Autodesk Inventor part; units mm, degrees
ref_plane "YZ Plane" through (0, 0, 0) normal (1, 0, 0) x (0, 1, 0)
ref_plane "XZ Plane" through (0, 0, 0) normal (0, 1, 0) x (-1, 0, 0)
ref_plane "XY Plane" through (0, 0, 0) normal (0, 0, 1) x (1, 0, 0)
sketch "Sketch1" plane through (0, 0, 0) normal (0, 0, 1) x (1, 0, 0)
  line L0 (-20, -20) -> (20, -20)
  line L1 (20, -20) -> (20, 20)
  line L2 (20, 20) -> (-20, 20)
  line L3 (-20, 20) -> (-20, -20)
  line L4 (-20, -20) -> (20, 20) construction
  line L5 (20, -20) -> (-20, 20) construction
  point P0 (0, 0)
  dimension "d0" = 40
  dimension "d1" = 40
extrude "Extrusion1" add sketch "Sketch1" along normal blind 10
sketch "Sketch2" plane through (0, 0, 10) normal (0, 0, 1) x (1, 0, 0)
  circle A0 centre (-14, 14) radius 1.05
  circle A1 centre (-14, -14) radius 1.05
  circle A2 centre (14, -14) radius 1.05
  circle A3 centre (14, 14) radius 1.05
  point P0 (0, 0)
  dimension "d4" = 2.1
  dimension "d5" = 2.1
  dimension "d6" = 2.1
  dimension "d7" = 2.1
  dimension "d8" = 14
  dimension "d9" = 14
  dimension "d10" = 14
  dimension "d11" = 14
extrude "Extrusion2" cut sketch "Sketch2" against normal blind 10
sketch "Sketch3" plane through (0, 0, 10) normal (0, 0, 1) x (1, 0, 0)
  line L0 (-7.5, -18) -> (7.5, -18)
  line L1 (7.5, -18) -> (7.5, -10)
  line L2 (7.5, -10) -> (-7.5, -10)
  line L3 (-7.5, -10) -> (-7.5, -18)
  line L4 (-7.5, -18) -> (7.5, -10) construction
  line L5 (7.5, -18) -> (-7.5, -10) construction
  point P0 (0, 0)
  point P1 (0, -14)
  dimension "d14" = 15
  dimension "d15" = 8
  dimension "d16" = 14
extrude "Extrusion3" cut sketch "Sketch3" against normal blind 10
sketch "Sketch4" plane through (-20, -20, 0) normal (0, -1, 0) x (1, 0, 0)
  line L0 (0, 0) -> (-10, 0)
  line L1 (-10, 0) -> (-10, 10)
  line L2 (-10, 10) -> (0, 10)
  line L3 (0, 10) -> (0, 0)
  line L4 (50, 0) -> (40, 0)
  line L5 (40, 0) -> (40, 10)
  line L6 (40, 10) -> (50, 10)
  line L7 (50, 10) -> (50, 0)
  line L8 (0, 0) -> (0, 10)
  line L9 (40, 0) -> (40, 10)
  line L10 (0, 0) -> (40, 0)
  line L11 (0, 10) -> (40, 10)
  point P0 (20, 0)
  dimension "d19" = 10
  dimension "d20" = 10
extrude "Extrusion4" add sketch "Sketch4" against normal blind 5 contours L0 L1 L2 L3 | L5 L6 L7 L4
sketch "Sketch5" plane through (-20, -15, 0) normal (0, 1, 0) x (1, 0, 0)
  circle A0 centre (-5, -5) radius 2.05
  circle A1 centre (45, -5) radius 2.05
  line L0 (-10, 0) -> (-10, -10)
  line L1 (-10, -10) -> (0, -10)
  line L2 (50, 0) -> (40, 0)
  line L3 (50, -10) -> (50, 0)
  point P0 (20, 0)
  dimension "d23" = 4.1
  dimension "d24" = 4.1
  dimension "d25" = 5
  dimension "d26" = 5
  dimension "d27" = 5
  dimension "d28" = 5
extrude "Extrusion5" cut sketch "Sketch5" against normal blind 5
sketch "Sketch6" plane through (-20, 20, 0) normal (0, 1, 0) x (1, 0, 0)
  line L0 (30, -10) -> (10, -10)
  line L1 (10, -10) -> (10, 0)
  line L2 (10, 0) -> (30, 0)
  line L3 (30, 0) -> (30, -10)
  line L4 (40, -10) -> (0, -10)
  line L5 (40, 0) -> (40, -10)
  line L6 (40, 0) -> (0, 0)
  line L7 (0, 0) -> (0, -10)
  point P0 (20, 0)
  dimension "d33" = 20
  dimension "d34" = 10
extrude "Extrusion6" add sketch "Sketch6" along normal blind 32 contours L0 L1 L2 L3
sketch "Sketch7" plane through (0, 0, 0) normal (0, 0, -1) x (-1, 0, 0)
  circle A0 centre (-7.5, 49.5) radius 1.05
  circle A1 centre (-7.5, 22.5) radius 1.05
  circle A2 centre (7.5, 49.5) radius 1.05
  circle A3 centre (7.5, 22.5) radius 1.05
  line L0 (-10, 52) -> (10, 52)
  line L1 (-10, 20) -> (-10, 52)
  point P0 (0, 0)
  dimension "d35" = 2.1
  dimension "d36" = 2.1
  dimension "d37" = 2.1
  dimension "d38" = 2.1
  dimension "d39" = 15
  dimension "d40" = 27
  dimension "d41" = 2.5
  dimension "d42" = 2.5
extrude "Extrusion7" cut sketch "Sketch7" against normal blind 32
properties part number "camera_new"
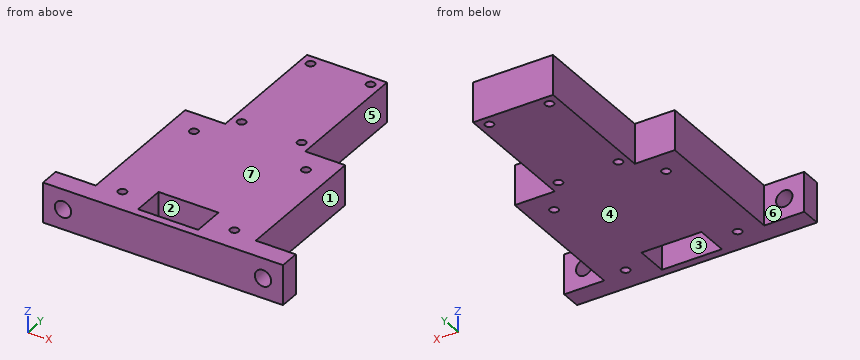
Design review of the part built by this model. Coordinates are the model's own, in mm. Face numbers are marked on the shaded views. A direction names the side the tool comes from. Round coordinates to 2 decimals unless told otherwise and drop trailing zeros. Write each loop counter-clockwise with the first axis right and the second up, starting at its lowest first coordinate (ties: lowest second). Pieces come first, ordered by that corner, then holes. Notation, with made-up numbers: M 85,-28 L 123,-28 A21 cw 123,3 Z; hole C 30,52.5 d5. An arc over 180 degrees is marked long. One line per item, written item: value. Start each with the question number.
1. Draft analysis for pull direction X (two halves, no side actions). For the marked faces 1, 2, 3 and 4, state which applies: pulls with the +X half, pulls with the -X half, needs draft (parallel to the pull), parting line crosses it, or undercut.
2. Take a section at A-A on z = 5. State how many separate pieces and enclosed holes the cut face has, then the cut area to 3 significant figures.
3. Take a section at B-B on y = 14. State the section outline as (x, z) points, then the cut area to 3 significant figures.
4. For the marked faces 5, 6 and 7, list the 3-axis set-ups (+Z, -Z, +X, -X, +Y, -Y) from which the entire face can be reached by the end or side of a thin tool; tool diameter is ignored.
5. To check wall thickness, follow probe 1 along X at (y, z) = (-17.4, 5); probe 2 along Y at (x, z) = (14, 5.5); probe 3 along Y at (x, z) = (3, 8.25). State the ranges of each line that lie inside material, in increasing order. Write a range as from..to.
6. Take a section at C-C on x = -1.5. State the section outline as (y, z) points.
7. Clearance check with flat-ended pins moving along their axes: P1, Ø5, axis at x = 25, z = 4, coming from the +Y side; P2, Ø5, axis at y = 28, z = 9, coming from the +X side; P3, Ø1.7, axis at x = 14, y = 14, coming from the -Z side; P4, Ø4, axis at y = 37, z = 2.5, coming from the -X side. State where each tip first meets the part, or that it passes through.
Computed:
1. face 1: pulls with the +X half
1. face 2: undercut
1. face 3: undercut
1. face 4: needs draft
2. separate pieces: 3
2. enclosed holes: 9
2. area: 2,150 mm²
3. outline: M -20,0 L -15.05,0 L -15.05,10 L -20,10 Z; M -12.95,0 L 12.95,0 L 12.95,10 L -12.95,10 Z; M 15.05,0 L 20,0 L 20,10 L 15.05,10 Z
3. area: 358 mm²
4. face 5: +Z, -Z, +X, +Y
4. face 6: +Z, -Z, -X, +Y
4. face 7: +Z, +X, -X, +Y, -Y
5. probe 1: x = -30..-27.05, -22.95..-7.5, 7.5..22.95, 27.05..30
5. probe 2: y = -20..-15.05, -12.95..12.95, 15.05..20
5. probe 3: y = -20..-18, -10..52
6. outline: M -20,0 L -18,0 L -18,10 L -20,10 Z; M -10,0 L 52,0 L 52,10 L -10,10 Z
7. P1: stops at y = -15
7. P2: stops at x = 10
7. P3: passes through
7. P4: stops at x = -10
